Work out the finished part from the listing and answer in its coordinate system (mm). A direction names the side the tool comes from. Round coordinates to 2 decimals unless told otherwise and drop trailing zeros. Write each loop counter-clockwise with the first axis right and the second up, starting at its lowest first coordinate (ties: lowest second). Pieces come first, ordered by that corner, then holes.
1. A tool of negligible diameter and unlimited length cuts with its end or side. For faces 1 (the face through (1.955, 10.669, 1.854)), 2 (the face through (7, 9.3, 8)), 3 (the face through (13, 1, 11)), from which of +Z, -Z, +X, -X, +Y, -Y can it reach the whole face along a straight path? Write none if from no direction.
2. Find section A-A (y = 7). Write down the section's boundary in (x, z), and give its area (3 significant figures).
3. Find section D-D (y = 11). Count the separate pieces of the cut face and the enclosed holes in it, and give its area (3 significant figures).
4. Find section C-C (z = 9.5). Write down the section's boundary in (x, y), and give its area (3 significant figures).
5. Find section B-B (x = 32). Write down the section's boundary in (y, z), and give its area (3 significant figures).
6. Straight lines are drawn through the part: probe 1 along Y at (x, z) = (12.5, 12); probe 2 along X at (y, z) = (7, 24); probe 3 along Z at (x, y) = (8.5, 0.5). For each, find the intervals that lie inside material, in ascending order.
7. Flat-ended cylindrical pins translate along their axes: pin 1 Ø3 at (y, z) = (10.5, 10) entering from +X; pin 2 Ø4.5 at (x, z) = (5.5, 21.5) entering from -Y; pin 3 Ø3.5 at (x, y) = (32, 7) entering from -Z. Find the tip coordinate at first contact, or state that the pin passes through.
8. Determine the mould class of faces 4 (the face through (13, 11, 11)), 5 (the face through (26, 6, 16)), 6 (the face through (21, 12, 17)), 7 (the face through (6.33, 6.5, 19.78)) for opening direction Y: pulls with the +Y half, pulls with the -Y half, needs draft (parallel to the pull), parting line crosses it, or undercut.
Autodesk Inventor part; units mm, degrees
ref_plane "YZ Plane" through (0, 0, 0) normal (1, 0, 0) x (0, 1, 0)
ref_plane "XZ Plane" through (0, 0, 0) normal (0, 1, 0) x (-1, 0, 0)
ref_plane "XY Plane" through (0, 0, 0) normal (0, 0, 1) x (1, 0, 0)
sketch "Sketch1" plane through (0, 0, 0) normal (0, 1, 0) x (-1, 0, 0)
  line L0 (0, 0) -> (0, 27)
  line L1 (0, 27) -> (-52, 27)
  line L2 (-52, 27) -> (-52, 16)
  line L3 (-52, 16) -> (-13, 16)
  line L4 (-13, 16) -> (-13, 0)
  line L5 (-13, 0) -> (0, 0)
  dimension "d0" = 27
  dimension "d1" = 52
  dimension "d2" = 11
  dimension "d3" = 39
  dimension "d57" = 16
extrude "Extrusion1" add sketch "Sketch1" along normal blind 12
sketch "Sketch2" plane through (0, 0, 0) normal (0, -1, 0) x (1, 0, 0)
  line L0 (0, 0) -> (0, 27)
  line L1 (0, 27) -> (52, 27)
  point P0 (5.5, 21.5)
  dimension "d6" = 5.5
  dimension "d7" = 5.5
hole "Hole1" at (5.5, 0, 21.5) direction (0, 1, 0) diameter 3.5 end through all counterbore diameter 8 counterbore depth 6.5
sketch "Sketch3" plane through (0, 12, 0) normal (0, 1, 0) x (1, 0, 0)
  line L0 (0, 0) -> (0, -27)
  line L1 (13, 0) -> (0, 0)
  point P0 (8, -5.5)
  dimension "d15" = 8
  dimension "d16" = 5.5
hole "Hole2" at (8, 12, 5.5) direction (0, -1, 0) diameter 2.459 end through all
sketch "Sketch4" plane through (13, 0, 16) normal (1, 0, 0) x (0, 0, -1)
  line L0 (0, 0) -> (0, 12)
  line L1 (16, 2.7) -> (0, 2.7)
  line L2 (0, 2.7) -> (0, 9.3)
  line L3 (0, 9.3) -> (16, 9.3)
  line L4 (16, 9.3) -> (16, 2.7)
  line L5 (0, 0) -> (16, 0)
  line L6 (0, 12) -> (16, 12)
  dimension "d58" = 12
  dimension "d59" = 6.6
  dimension "d60" = 2.7
extrude "Extrusion2" cut sketch "Sketch4" against normal through all
sketch "Sketch5" plane through (0, 0, 27) normal (0, 0, 1) x (1, 0, 0)
  line L0 (0, 0) -> (52, 0)
  line L1 (0, 0) -> (0, 12)
  point P0 (15.5, 7)
  dimension "d28" = 7
  dimension "d29" = 15.5
hole "Hole3" at (15.5, 7, 27) direction (0, 0, -1) diameter 4.917 end through all
sketch "Sketch6" plane through (0, 0, 27) normal (0, 0, 1) x (1, 0, 0)
  line L0 (0, 0) -> (52, 0)
  line L1 (0, 0) -> (0, 12)
  point P0 (32, 7)
  dimension "d37" = 7
  dimension "d38" = 32
hole "Hole4" at (32, 7, 27) direction (0, 0, -1) diameter 3.242 end through all
sketch "Sketch7" plane through (0, 0, 0) normal (0, -1, 0) x (1, 0, 0)
  line L0 (0, 27) -> (52, 27)
  point P0 (0, 0)
hole "Hole5" at (52, 0, 27) direction (0, 1, 0) diameter 19 end through all
fillet "Fillet1" radius 1.5 2 edges at (42.5, 6, 27) (52, 6, 17.5)
fillet "Fillet2" radius 6.5 4 edges at (13, 1.35, 0) (13, 10.65, 0) (0, 10.65, 0) (0, 1.35, 0)
fillet "Fillet3" radius 1 1 edges at (0, 6, 27)
fillet "Fillet4" radius 1 2 edges at (13, 1.35, 16) (13, 10.65, 16)
equation "\"d60\" = -0.5 * d59 + 0.5 * d58"
Worked answers:
1. face 1: -Z, -X, +Y, -Y
1. face 2: -Z, +X, -X
1. face 3: -Z, +X, +Y, -Y
2. outline: (0, 16) - (13.04, 16) - (13.04, 27) - (1, 27) arc R1 ccw to (0, 26) - close; (17.96, 16) - (30.38, 16) - (30.38, 27) - (17.96, 27) - close; (33.62, 16) - (52, 16) - (52, 16.1) arc R1.5 ccw to (50.7, 17.59) arc R9.5 cw to (42.59, 25.7) arc R1.5 ccw to (41.1, 27) - (33.62, 27) - close; hole circle Ø3.5 at (5.5, 21.5)
2. area: 401 mm2
3. separate pieces: 1
3. enclosed holes: 2
3. area: 676 mm2
4. outline: (0, 0) - (13, 0) - (13, 2.7) - (0, 2.7) - close; (0, 9.3) - (13, 9.3) - (13, 12) - (0, 12) - close
4. area: 70.2 mm2
5. outline: (0, 16) - (5.38, 16) - (5.38, 27) - (0, 27) - close; (8.62, 16) - (12, 16) - (12, 27) - (8.62, 27) - close
5. area: 96.3 mm2
6. probe 1: y = 0 to 2.7, 9.3 to 12
6. probe 2: x = 0 to 13.04, 17.96 to 30.38, 33.62 to 42.99
6. probe 3: z = 0.32 to 4.38, 6.62 to 18.85, 24.15 to 27
7. pin 1: stops at x = 13
7. pin 2: stops at y = 6.5
7. pin 3: stops at z = 16
8. face 4: needs draft
8. face 5: undercut
8. face 6: pulls with the +Y half
8. face 7: pulls with the -Y half
